Build history of the part. All positions in model axes, mm. A direction names the side the tool comes from. Round coordinates to 2 decimals unless told otherwise and drop trailing zeros. Write each loop counter-clockwise with the first axis right and the second up, starting at its lowest first coordinate (ties: lowest second). Pieces come first, ordered by that corner, then holes.
1) Flat gauge pins, fed straight in: pin 1 (11.5 mm diameter, centred on x = 232, y = -8.5, fed in from +Z); pin 2 (10.5 mm diameter, centred on y = 1, z = 5, fed in from -X); pin 3 (3 mm diameter, centred on y = 4.5, z = 3, fed in from +X). Where does each tip first touch, or does it go through?
2) Saw through at C-C (z = 3.5). Write the cut outline in (x, y), plus the area to 3 significant figures.
3) Saw through at B-B (x = -217). Write the cut outline in (y, z) (3 decimals), plus the area to 3 significant figures.
4) Saw through at A-A (y = -8.5). Write the cut outline in (x, z) (1 decimal).
5) Wall check: probe 1 along X at (y, z) = (15, 8.75); probe 2 along Z at (x, y) = (248, -9) (3 decimals). Give the ranges that are in metal, low to high.
6) Which spindle directions (+Z, -Z, +X, -X, +Y, -Y) get a long thin tool onto all of the face, cutting with end or side? Do faces 1 (the flat face through (204.788, 0, 5)), 2 (the flat face through (-204.788, 0, 5)), 3 (the flat face through (20, 19.05, 0)). Say none if no direction does.
from build123d import *

# Parameters (mm, degrees)
F0_W     = 409.575
F0_H     = 38.1
F1_DEPTH = 9.525
F2_W     = 50.8
F2_H     = 38.1
F2_W_2   = 98.425
F3_DEPTH = 9.525


with BuildPart() as f1:
    # F0 (on Top) → F1 (new body, symmetric)
    with BuildSketch(Plane.XY):
        Rectangle(F0_W, F0_H)
    extrude(amount=F1_DEPTH, both=True)

    # F2 (on Top) → F3 (join, through all)
    with BuildSketch(Plane.XY):
        with Locations((-230.1875, 0)):
            Rectangle(F2_W, F2_H)
        with Locations((254, 0)):
            Rectangle(F2_W_2, F2_H)
    extrude(amount=-F3_DEPTH)


solid = f1.part
Evaluation:
1. pin 1: stops at z = 0
1. pin 2: stops at x = -255.59
1. pin 3: stops at x = 204.79
2. outline: (-204.79, -19.05) - (204.79, -19.05) - (204.79, 19.05) - (-204.79, 19.05) - close
2. area: 15,600 mm2
3. outline: (-19.05, -9.525) - (19.05, -9.525) - (19.05, 0) - (-19.05, 0) - close
3. area: 363 mm2
4. outline: (-255.6, -9.5) - (303.2, -9.5) - (303.2, 0) - (204.8, 0) - (204.8, 9.5) - (-204.8, 9.5) - (-204.8, 0) - (-255.6, 0) - close
5. probe 1: x = -204.79 to 204.79
5. probe 2: z = -9.525 to 0
6. face 1: +Z, +X, +Y, -Y
6. face 2: +Z, -X, +Y, -Y
6. face 3: +Z, -Z, +X, -X, +Y
